from build123d import *

# Parameters (mm, degrees)
EXTRUDE_1_DEPTH          = 200
CUT_EXTRUDE_1_REACH      = 203.99
SKETCH_2_R               = 1.75
MIRROR_2_COPY_1_REACH    = 203.99
MIRROR_2_COPY_1_SKETCH_R = 1.75


with BuildPart() as part:
    # Эскиз1 → Бобышка-Вытянуть1 (new body)
    with BuildSketch(Plane(origin=(0, 0, 0), x_dir=(1, 0, 0), z_dir=(0, 1, 0))):
        Polygon((0, 0), (20, 0), (20, 1.5), (1.5, 1.5), (1.5, 20), (0, 20), align=None)
    extrude(amount=EXTRUDE_1_DEPTH)

    # Эскиз2 → Вырез-Вытянуть1 (cut, up to next)
    with BuildSketch(Plane.XY, mode=Mode.PRIVATE) as cut_extrude_1_sk1:
        with Locations((10, 190)):
            Circle(SKETCH_2_R)
    cut_extrude_1_tool1 = extrude(cut_extrude_1_sk1.sketch, amount=-CUT_EXTRUDE_1_REACH, mode=Mode.PRIVATE) & part.part
    cut_extrude_1 = cut_extrude_1_tool1.solids().sort_by_distance((10, 190, 0))[0]
    add(cut_extrude_1, mode=Mode.SUBTRACT)

    # Зеркальное отражение1: Вырез-Вытянуть1 across plane
    add(cut_extrude_1.mirror(Plane(origin=(0, 0, 0), x_dir=(-0.7071067811865482, 0, 0.7071067811865468), z_dir=(-0.7071067811865468, 0, -0.7071067811865482))), mode=Mode.SUBTRACT)

    # Зеркальное отражение2: Вырез-Вытянуть1 across plane
    add(cut_extrude_1.mirror(Plane(origin=(0, 100, 0), x_dir=(0, 0, 1), z_dir=(0, -1, 0))), mode=Mode.SUBTRACT)

    # Зеркальное отражение2 copy 1 sketch → Зеркальное отражение2 copy 1 (cut, up to next)
    with BuildSketch(Plane(origin=(0, 200, 0), x_dir=(0, 0, -1), z_dir=(-1, 0, 0)), mode=Mode.PRIVATE) as mirror_2_copy_1_sk1:
        with Locations((10, 190)):
            Circle(MIRROR_2_COPY_1_SKETCH_R)
    mirror_2_copy_1_tool1 = extrude(mirror_2_copy_1_sk1.sketch, amount=-MIRROR_2_COPY_1_REACH, mode=Mode.PRIVATE) & part.part
    add(mirror_2_copy_1_tool1.solids().sort_by_distance((0, 10, -10))[0], mode=Mode.SUBTRACT)


solid = part.part
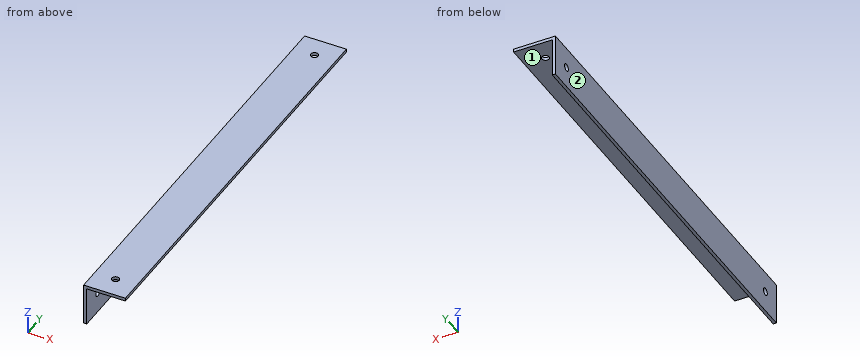
Part model, mm, in its own coordinate system. Face numbers are marked on the shaded views. A direction names the side the tool comes from. Give positions to 0.01 mm unless a question says otherwise; leave off trailing zeros. Write each loop counter-clockwise with the first axis right and the second up, starting at its lowest first coordinate (ties: lowest second). Pieces come first, ordered by that corner, then holes.
1) Probe L1, parallel to Y at x = 0.35, z = -10; L2, parallel to X at y = 190, z = -0.5; L3, parallel to Z at x = 0.65, y = 10. List the from-to ranges inside material, lowest first.
Resolved:
L1: y = 0 to 8.25, 11.75 to 188.25, 191.75 to 200
L2: x = 0 to 8.25, 11.75 to 20
L3: z = -20 to -11.75, -8.25 to 0
2) Which spindle directions (+Z, -Z, +X, -X, +Y, -Y) get a long thin tool onto all of the face, cutting with end or side? Do the marked faces 1 and 2. Say none if no direction does.
Resolved:
face 1: -Z, +X, +Y, -Y
face 2: +Z, -Z, -X, +Y, -Y
3) Cut at C-C on y = 190. Write the cut outline in (x, z), then the cut area to 4 significant figures.
Resolved:
outline: (0, -20) - (1.5, -20) - (1.5, -11.75) - (0, -11.75) - close; (0, -8.25) - (1.5, -8.25) - (1.5, -1.5) - (8.25, -1.5) - (8.25, 0) - (0, 0) - close; (11.75, -1.5) - (20, -1.5) - (20, 0) - (11.75, 0) - close
area: 47.25 mm2
4) Cut at D-D on y = 146.5. Write the cut outline in (x, z).
Resolved:
outline: (0, -20) - (1.5, -20) - (1.5, -1.5) - (20, -1.5) - (20, 0) - (0, 0) - close
5) Pin check, flat tips, straight feed: pin 1 (4.5 mm diameter, centred on y = 10, z = -10, fed in from +X); pin 2 (5 mm diameter, centred on x = 13.5, y = 179.5, fed in from -Z); pin 3 (3 mm diameter, centred on x = 10, y = 10, fed in from +Z). Stop position of each tip, or through.
Resolved:
pin 1: stops at x = 1.5
pin 2: stops at z = -1.5
pin 3: passes through
6) Cut at A-A on z = -10. Write the cut outline in (x, y), then the cut area to 4 significant figures.
Resolved:
outline: (0, 0) - (1.5, 0) - (1.5, 8.25) - (0, 8.25) - close; (0, 11.75) - (1.5, 11.75) - (1.5, 188.25) - (0, 188.25) - close; (0, 191.75) - (1.5, 191.75) - (1.5, 200) - (0, 200) - close
area: 289.5 mm2
7) Cut at B-B on x = 10. Write the cut outline in (y, z).
Resolved:
outline: (0, -1.5) - (8.25, -1.5) - (8.25, 0) - (0, 0) - close; (11.75, -1.5) - (188.25, -1.5) - (188.25, 0) - (11.75, 0) - close; (191.75, -1.5) - (200, -1.5) - (200, 0) - (191.75, 0) - close
